from build123d import *

# Parameters (mm, degrees)
SKETCH1_R           = 1.75
BOSS_EXTRUDE1_DEPTH = 4
BOSS_EXTRUDE2_START = -4
BOSS_EXTRUDE2_DEPTH = 4


with BuildPart() as part:
    # Sketch1 → Boss-Extrude1 (new body)
    with BuildSketch(Plane(origin=(0, 0, 0), x_dir=(1, 0, 0), z_dir=(0, 1, 0))):
        with BuildLine():
            Line((30.75, 4), (11.409123542, 4))
            ThreePointArc((11.409123542, 4), (-12.09, 0), (11.409123542, -4))
            Line((11.409123542, -4), (30.75, -4))
            ThreePointArc((30.75, -4), (34.75, 0), (30.75, 4))
        make_face()
        with Locations(Location((30.75, 0, 0), (0, 0, 270))):
            Circle(SKETCH1_R, mode=Mode.SUBTRACT)
        with Locations(Location((0, 0, 0), (0, 0, 270))):
            Circle(SKETCH1_R, mode=Mode.SUBTRACT)
    extrude(amount=BOSS_EXTRUDE1_DEPTH)

    # Sketch2 → Boss-Extrude2 (add)
    with BuildSketch(Plane(origin=(0, 4, 0), x_dir=(1, 0, 0), z_dir=(0, 1, 0)).offset(BOSS_EXTRUDE2_START)):
        with BuildLine():
            ThreePointArc((13.631289382, 5.312706446), (13.515656169, 5.600351625), (13.393953907, 5.885482032))
            ThreePointArc((13.393953907, 5.885482032), (12.042056289, 5.896469103), (10.729798038, 5.571313495))
            ThreePointArc((10.729798038, 5.571313495), (11.16927846, 4.627668819), (11.525956115, 3.649717201))
            ThreePointArc((11.525956115, 3.649717201), (12.683545875, 4.348379847), (13.631289382, 5.312706446))
        make_face()
        with BuildLine():
            ThreePointArc((0.54, 12.077934426), (0.914536108, 13.376961211), (1.6, 14.542245356))
            ThreePointArc((1.6, 14.542245356), (1.907781307, 14.505077404), (2.214705946, 14.461396114))
            ThreePointArc((2.214705946, 14.461396114), (2.575965524, 13.158462861), (2.602230245, 11.806629399))
            ThreePointArc((2.602230245, 11.806629399), (1.576960473, 11.986713297), (0.54, 12.077934426))
        make_face()
        with BuildLine():
            ThreePointArc((5.882126404, 13.395427913), (5.89385242, 12.043390174), (5.569341946, 10.73082151))
            ThreePointArc((5.569341946, 10.73082151), (4.625616537, 11.170128542), (3.647599401, 11.526626506))
            ThreePointArc((3.647599401, 11.526626506), (4.345586373, 12.684452949), (5.309291379, 13.63261989))
            ThreePointArc((5.309291379, 13.63261989), (5.596965518, 13.51705874), (5.882126404, 13.395427913))
        make_face()
        with BuildLine():
            ThreePointArc((9.148689668, 11.416583436), (8.810083014, 10.10758035), (8.156912198, 8.92372587))
            ThreePointArc((8.156912198, 8.92372587), (7.359044479, 9.592317987), (6.506620931, 10.189798038))
            ThreePointArc((6.506620931, 10.189798038), (7.480492108, 11.12752018), (8.656763324, 11.793953907))
            ThreePointArc((8.656763324, 11.793953907), (8.904725778, 11.607874862), (9.148689668, 11.416583436))
        make_face()
        with BuildLine():
            ThreePointArc((11.791784851, 8.659717665), (11.125921009, 7.482955629), (10.188602363, 6.508493058))
            ThreePointArc((10.188602363, 6.508493058), (9.5909657, 7.360806813), (8.922226997, 8.158551674))
            ThreePointArc((8.922226997, 8.158551674), (10.105614668, 8.8122653), (11.414291155, 9.151549455))
            ThreePointArc((11.414291155, 9.151549455), (11.605643693, 8.907633495), (11.791784851, 8.659717665))
        make_face()
        with BuildLine():
            ThreePointArc((-1.603643062, 14.541844069), (-1.911415048, 14.504599013), (-2.218328735, 14.460840834))
            ThreePointArc((-2.218328735, 14.460840834), (-2.578838281, 13.157851673), (-2.604399509, 11.806151075))
            ThreePointArc((-2.604399509, 11.806151075), (-1.579162842, 11.98642335), (-0.542219148, 12.077835005))
            ThreePointArc((-0.542219148, 12.077835005), (-0.917469165, 13.376808049), (-1.603643062, 14.541844069))
        make_face()
        with BuildLine():
            ThreePointArc((-5.312706446, 13.631289382), (-5.600351625, 13.515656169), (-5.885482032, 13.393953907))
            ThreePointArc((-5.885482032, 13.393953907), (-5.896469103, 12.042056289), (-5.571313495, 10.729798038))
            ThreePointArc((-5.571313495, 10.729798038), (-4.627668819, 11.16927846), (-3.649717201, 11.525956115))
            ThreePointArc((-3.649717201, 11.525956115), (-4.348379847, 12.683545875), (-5.312706446, 13.631289382))
        make_face()
        with BuildLine():
            ThreePointArc((-8.659717665, 11.791784851), (-8.907633495, 11.605643693), (-9.151549455, 11.414291155))
            ThreePointArc((-9.151549455, 11.414291155), (-8.8122653, 10.105614668), (-8.158551674, 8.922226997))
            ThreePointArc((-8.158551674, 8.922226997), (-7.360806813, 9.5909657), (-6.508493058, 10.188602363))
            ThreePointArc((-6.508493058, 10.188602363), (-7.482955629, 11.125921009), (-8.659717665, 11.791784851))
        make_face()
        with BuildLine():
            ThreePointArc((-11.416583436, 9.148689668), (-11.607874862, 8.904725778), (-11.793953907, 8.656763324))
            ThreePointArc((-11.793953907, 8.656763324), (-11.12752018, 7.480492108), (-10.189798038, 6.506620931))
            ThreePointArc((-10.189798038, 6.506620931), (-9.592317987, 7.359044479), (-8.92372587, 8.156912198))
            ThreePointArc((-8.92372587, 8.156912198), (-10.10758035, 8.810083014), (-11.416583436, 9.148689668))
        make_face()
        with BuildLine():
            ThreePointArc((-13.395427913, 5.882126404), (-13.51705874, 5.596965518), (-13.63261989, 5.309291379))
            ThreePointArc((-13.63261989, 5.309291379), (-12.684452949, 4.345586373), (-11.526626506, 3.647599401))
            ThreePointArc((-11.526626506, 3.647599401), (-11.170128542, 4.625616537), (-10.73082151, 5.569341946))
            ThreePointArc((-10.73082151, 5.569341946), (-12.043390174, 5.89385242), (-13.395427913, 5.882126404))
        make_face()
        with BuildLine():
            ThreePointArc((-14.461396114, 2.214705946), (-14.505077404, 1.907781307), (-14.542245356, 1.6))
            ThreePointArc((-14.542245356, 1.6), (-13.376961211, 0.914536108), (-12.077934426, 0.54))
            ThreePointArc((-12.077934426, 0.54), (-11.986713297, 1.576960473), (-11.806629399, 2.602230245))
            ThreePointArc((-11.806629399, 2.602230245), (-13.158462861, 2.575965524), (-14.461396114, 2.214705946))
        make_face()
    extrude(amount=BOSS_EXTRUDE2_DEPTH)


solid = part.part
Build history of the part. All positions in model axes, mm. A direction names the side the tool comes from. Give positions to 0.01 mm unless a question says otherwise; leave off trailing zeros. Order: outer loops, then holes, each group sorted by start corner. A loop starts at its lowest first (then second) coordinate and runs counter-clockwise, first axis right, second up. Notation, with made-up numbers: M 34,38 L 85,38 A34 cw 85,76 Z; hole C -22.75,6.25 d1. An arc over 180 degrees is marked long. Use one line per item in the form item = value.
Q1. Pull direction X, two halves, no side cores. Call faces 1 (the cylindrical face through (0.01, 1.97, -12.09)), 2 (the cylindrical face through (34.75, 1.97, 0.09)), 3 (the cylindrical face through (-12.7, 1.97, -4.36)), 4 (the cylindrical face through (0.907, 1.972, -13.36)): released by +X, released by -X, zero draft, split by the parting line, or undercut.
Conclusion:
face_1 = undercut
face_2 = released by +X
face_3 = released by -X
face_4 = undercut
Q2. Slice it at C-C, the plane y = 3.45. State how many separate pieces and enclosed holes the cut face has, and give its area (3 significant figures).
Conclusion:
separate_pieces = 1
enclosed_holes = 2
area = 660 mm2
Q3. Which spindle directions (+Z, -Z, +X, -X, +Y, -Y) get a long thin tool onto all of the face, cutting with end or side? Do faces 5 (the cylindrical face through (5.9, 2, -12.1)), 6 (the cylindrical face through (-0.91, 1.97, -13.36)), 7 (the flat face through (21, 2, 4)). Say none if no direction does.
Conclusion:
face_5 = +Y, -Y
face_6 = -Z, +Y, -Y
face_7 = +Z, +X, +Y, -Y
Q4. Slice it at A-A, the plane x = 0. Write the cut outline in (y, z), and give its area (3 significant figures).
Conclusion:
outline = M 0,-12.09 L 4,-12.09 L 4,-1.75 L 0,-1.75 Z; M 0,1.75 L 4,1.75 L 4,12.09 L 0,12.09 Z
area = 82.7 mm2
Q5. Wall check: probe 1 along X at (y, z) = (1.85, 0); probe 2 along X at (y, z) = (1, 1.25); probe 3 along Z at (x, y) = (12, 0.5). Give the ranges that are in metal, low to high.
Conclusion:
probe_1 = -12.09 to -1.75, 1.75 to 29, 32.5 to 34.75
probe_2 = -12.03 to -1.22, 1.22 to 29.53, 31.97 to 34.55
probe_3 = -5.89 to 4
Q6. Pin check, flat tips, straight feed: P1, Ø3, axis at x = 0, z = 0, coming from the -Y side; P2, Ø1.5, axis at x = 15.5, y = 1, coming from the -Z side; P3, Ø1, axis at x = 11, y = 2, coming from the +Z side. Stop position of each tip, or through.
Conclusion:
P1 = through
P2 = -4
P3 = 5.99
Q7. Slice it at D-D, the plane x = 27.5. Write the cut outline in (y, z), and give its area (3 significant figures).
Conclusion:
outline = M 0,-4 L 4,-4 L 4,4 L 0,4 Z
area = 32.0 mm2
Q8. Slice it at B-B, the plane z = 0. Write the cut outline in (x, y).
Conclusion:
outline = M -12.09,0 L -1.75,0 L -1.75,4 L -12.09,4 Z; M 1.75,0 L 29,0 L 29,4 L 1.75,4 Z; M 32.5,0 L 34.75,0 L 34.75,4 L 32.5,4 Z
